```python
from build123d import *

# Parameters (mm, degrees)
SKETCH1_W                = 154.432
SKETCH1_H                = 99.822
BOSS_EXTRUDE1_DEPTH      = 15.6845
BOSS_EXTRUDE2_DEPTH      = 10.16
BOSS_EXTRUDE2_DEPTH_BACK = 164.592
SKETCH2_R                = 3.048
SKETCH2_3_R              = 3.048
BOSS_EXTRUDE3_DEPTH      = 10.16
SKETCH3_R                = 1.651
CUT_EXTRUDE1_DEPTH       = 102.841429866


with BuildPart() as part:
    # Sketch1 → Boss-Extrude1 (new body)
    with BuildSketch(Plane.XY):
        Rectangle(SKETCH1_W, SKETCH1_H)
    extrude(amount=BOSS_EXTRUDE1_DEPTH)

    # Sketch2 → Boss-Extrude2 (add, two sides: drawn at the far end of the back side and taken through both)
    with BuildSketch(Plane.ZY.offset(77.216).offset(-BOSS_EXTRUDE2_DEPTH_BACK)):
        with Locations((7.84225, 34.417)):
            Circle(SKETCH2_R)
        with Locations((7.84225, 11.557)):
            Circle(SKETCH2_R)
        with Locations((7.84225, -34.163)):
            Circle(SKETCH2_R)
    extrude(amount=BOSS_EXTRUDE2_DEPTH + BOSS_EXTRUDE2_DEPTH_BACK)

    # Sketch2<3> → Boss-Extrude3 (add)
    with BuildSketch(Plane.ZY.offset(77.216)):
        with Locations(Location((7.84225, -11.303, 0), (0, 0, 180))):
            Circle(SKETCH2_3_R)
    extrude(amount=BOSS_EXTRUDE3_DEPTH)

    # Sketch3 → Cut-Extrude1 (cut, through all)
    with BuildSketch(Plane.XY):
        with Locations((-62.6618, 46.609)):
            Circle(SKETCH3_R)
        with Locations((-62.6618, -46.609)):
            Circle(SKETCH3_R)
        with Locations((56.6928, -46.609)):
            Circle(SKETCH3_R)
        with Locations((56.6928, 46.609)):
            Circle(SKETCH3_R)
    extrude(amount=CUT_EXTRUDE1_DEPTH, mode=Mode.SUBTRACT)


solid = part.part
```
Can you work these out from the model? Positions are in its coordinate system, mm. A direction names the side the tool comes from. Give positions to 0.01 mm unless a question says otherwise; leave off trailing zeros. Write each loop counter-clockwise with the first axis right and the second up, starting at its lowest first coordinate (ties: lowest second). Pieces come first, ordered by that corner, then holes. Notation, with made-up numbers: (35.5, 25) -> (82.5, 25) arc R27 ccw to (82.5, 42) -> close; hole circle Ø3 at (-23, 59.25). An arc over 180 degrees is marked (long way). One line per item, written item: value.
Q1. Which directions (+Z, -Z, +X, -X, +Y, -Y) give clear straight access to the entire face, cutting with the end or side of a thin tool? Please do faces 3 (the face through (-82.225, -8.599, 6.436)), 4 (the face through (87.376, 12, 8)), 5 (the face through (82.37, -31.14, 7.45)).
Results found:
face 3: -X
face 4: +Z, -Z, +X, +Y, -Y
face 5: +X
Q2. Imagine slicing it at A-A on y = 29. Please give me the cut outline in (x, z), and give its area (3 significant figures).
Results found:
outline: (-77.22, 0) -> (77.22, 0) -> (77.22, 15.68) -> (-77.22, 15.68) -> close
area: 2,420 mm^2
Q3. Imagine slicing it at B-B on z = 9. Give the number of separate pieces and of enclosed holes in the cut face, and give its area (3 significant figures).
Results found:
separate pieces: 1
enclosed holes: 4
area: 15,800 mm^2
Q4. Please list where these lines run through material, in increasing order: line 1 (X direction, y = 46, z = 12.75); line 2 (X direction, y = -2, z = 6). Write a range as [from, to].
Results found:
line 1: x = [-77.22, -64.2], [-61.13, 55.16], [58.23, 77.22]
line 2: x = [-77.22, 77.22]
Q5. We'd pull the mould along Y, two halves only. Please class faces 1 (the face through (-82.225, 9.702, 5.423)), 2 (the face through (-87.376, -34, 8)): +Y half, -Y half, draft (parallel to the pull), parting line (faces both ways), or undercut.
Results found:
face 1: undercut
face 2: draft
Q6. For P1, Ø5, axis at y = 26, z = 12, coming from the +X side; P2, Ø2, axis at x = -62.66, y = 46.61, coming from the -Z side; P3, Ø2, axis at y = -14.5, z = 12, coming from the -X side, each with a flat end and sliding along its axis, tell me the tip position at first contact or that it passes through.
Results found:
P1: stops at x = 77.22
P2: passes through
P3: stops at x = -77.22
